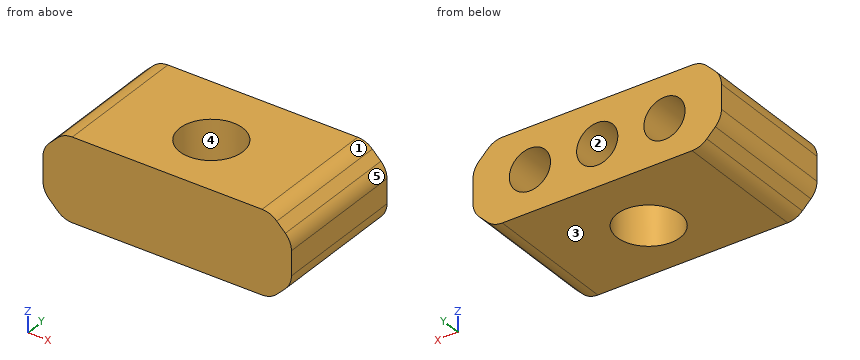
from build123d import *

# Parameters (mm, degrees)
SKETCH1_W                = 24
SKETCH1_H                = 13
BOSS_EXTRUDE1_DEPTH      = 4
BOSS_EXTRUDE1_DEPTH_BACK = 4
SKETCH3_R                = 3.04
CUT_EXTRUDE1_DEPTH       = 7
CUT_EXTRUDE1_DEPTH_BACK  = 7
SKETCH4_R                = 1.99
CUT_EXTRUDE2_DEPTH       = 10
SKETCH5_R                = 1.99
CUT_EXTRUDE4_DEPTH       = 3.9
CHAMFER1_SIZE            = 2
FILLET1_R                = 2


with BuildPart() as part:
    # Sketch1 → Boss-Extrude1 (new body, two sides)
    with BuildSketch(Plane.XY) as boss_extrude1_sk:
        Rectangle(SKETCH1_W, SKETCH1_H)
    extrude(amount=BOSS_EXTRUDE1_DEPTH)
    extrude(boss_extrude1_sk.sketch, amount=-BOSS_EXTRUDE1_DEPTH_BACK)

    # Sketch3 → Cut-Extrude1 (cut, two sides)
    with BuildSketch(Plane.XY) as cut_extrude1_sk:
        with Locations((0, -0.5)):
            Circle(SKETCH3_R)
    extrude(amount=CUT_EXTRUDE1_DEPTH, mode=Mode.SUBTRACT)
    extrude(cut_extrude1_sk.sketch, amount=-CUT_EXTRUDE1_DEPTH_BACK, mode=Mode.SUBTRACT)

    # Sketch4 → Cut-Extrude2 (cut)
    with BuildSketch(Plane(origin=(0, 6.5, 0), x_dir=(1, 0, 0), z_dir=(0, 1, 0))):
        with Locations((-6.5, 0)):
            Circle(SKETCH4_R)
        with Locations((6.5, 0)):
            Circle(SKETCH4_R)
    extrude(amount=-CUT_EXTRUDE2_DEPTH, mode=Mode.SUBTRACT)

    # Sketch5 → Cut-Extrude4 (cut)
    with BuildSketch(Plane(origin=(0, 6.5, 0), x_dir=(1, 0, 0), z_dir=(0, 1, 0))):
        Circle(SKETCH5_R)
    extrude(amount=-CUT_EXTRUDE4_DEPTH, mode=Mode.SUBTRACT)

    # Chamfer1
    chamfer1_edges = [part.edges().sort_by_distance(p)[0] for p in [
        (12, 0, -4),
        (-12, 0, 4),
        (12, 0, 4),
        (-12, 0, -4),
    ]]
    chamfer(chamfer1_edges, length=CHAMFER1_SIZE)

    # Fillet1
    fillet1_edges = [part.edges().sort_by_distance(p)[0] for p in [
        (-10, 0, 4),
        (10, 0, 4),
        (12, 0, -2),
        (12, 0, 2),
        (-10, 0, -4),
        (10, 0, -4),
        (-12, 0, -2),
        (-12, 0, 2),
    ]]
    fillet(fillet1_edges, radius=FILLET1_R)


solid = part.part
For this review, take the finished solid that the model builds, in its own axes (mm). Face numbers are marked on the shaded views. A direction names the side the tool comes from. Round coordinates to 2 decimals unless told otherwise and drop trailing zeros. Order: outer loops, then holes, each group sorted by start corner. A loop starts at its lowest first (then second) coordinate and runs counter-clockwise, first axis right, second up. Notation, with made-up numbers: M 20.25,41.5 L 40.25,41.5 A23 ccw 40.25,77.5 Z; hole C 50.25,86.25 d6. An arc over 180 degrees is marked long. Write each question's results on one line, items separated by ' | '. Start each with the question number.
1. Add section C-C (y = -5.5). State the section outline as (x, z) points, then the cut area to 3 significant figures.
2. To check wall thickness, follow L1, parallel to X at y = 3.55, z = 0; L2, parallel to Z at x = -6.5, y = 2.5; L3, parallel to X at y = -0.5, z = 0.5. State the ranges of each line that lie inside material, in increasing order. Write a range as [from, to].
3. Tool access review of the marked faces 1 and 2: name each direction out of +Z, -Z, +X, -X, +Y, -Y from which nothing blocks a thin tool from reaching the whole face with its end or side.
4. Add section A-A (y = -0.5). State the section outline as (x, z) points, then the cut area to 3 significant figures.
5. Add section D-D (z = -1.75). State the section outline as (x, y) points, then the cut area to 3 significant figures.
6. Add section B-B (x = 0). State the section outline as (y, z) points.
7. Clearance check with flat-ended pins moving along their axes: pin 1 Ø1.2 at (x, z) = (-6, -0.5) entering from +Y; pin 2 Ø2 at (x, z) = (0, 0.5) entering from +Y. State where each tip first meets the part, or that it passes through.
8. Draft analysis for pull direction X (two halves, no side actions). For the marked faces 3, 4 and 5, state which applies: pulls with the +X half, pulls with the -X half, needs draft (parallel to the pull), parting line crosses it, or undercut.
Output values:
1) outline: M -12,-1.17 A2 ccw -11.41,-2.59 L -10.59,-3.41 A2 ccw -9.17,-4 L 9.17,-4 A2 ccw 10.59,-3.41 L 11.41,-2.59 A2 ccw 12,-1.17 L 12,1.17 A2 ccw 11.41,2.59 L 10.59,3.41 A2 ccw 9.17,4 L -9.17,4 A2 ccw -10.59,3.41 L -11.41,2.59 A2 ccw -12,1.17 Z | area: 183 mm^2
2) L1: [-12, -8.49], [-4.51, -1.99], [1.99, 4.51], [8.49, 12] | L2: [-4, -1.99], [1.99, 4] | L3: [-12, -8.43], [-4.57, -3.04], [3.04, 4.57], [8.43, 12]
3) face 1: +Z, +X, +Y, -Y | face 2: +Y
4) outline: M -12,-1.17 A2 ccw -11.41,-2.59 L -10.59,-3.41 A2 ccw -9.17,-4 L -3.04,-4 L -3.04,4 L -9.17,4 A2 ccw -10.59,3.41 L -11.41,2.59 A2 ccw -12,1.17 Z; M 3.04,-4 L 9.17,-4 A2 ccw 10.59,-3.41 L 11.41,-2.59 A2 ccw 12,-1.17 L 12,1.17 A2 ccw 11.41,2.59 L 10.59,3.41 A2 ccw 9.17,4 L 3.04,4 Z; hole C -6.5,0 d3.98; hole C 6.5,0 d3.98 | area: 110 mm^2
5) outline: M -11.91,-6.5 L 11.91,-6.5 L 11.91,6.5 L 7.45,6.5 L 7.45,-3.5 L 5.55,-3.5 L 5.55,6.5 L 0.95,6.5 L 0.95,2.6 L -0.95,2.6 L -0.95,6.5 L -5.55,6.5 L -5.55,-3.5 L -7.45,-3.5 L -7.45,6.5 L -11.91,6.5 Z; hole C 0,-0.5 d6.08 | area: 235 mm^2
6) outline: M -6.5,-4 L -3.54,-4 L -3.54,4 L -6.5,4 Z; M 2.54,-4 L 6.5,-4 L 6.5,-1.99 L 2.6,-1.99 L 2.6,1.99 L 6.5,1.99 L 6.5,4 L 2.54,4 Z
7) pin 1: y = -3.5 | pin 2: y = 2.6
8) face 3: needs draft | face 4: undercut | face 5: pulls with the +X half
